The model under review builds one solid part; all positions refer to its coordinate system, in mm. A direction names the side the tool comes from. Coordinates: 2 decimals unless noted, no trailing zeros. Loops run counter-clockwise (first coordinate to the right, second up) from the corner with the lowest first, then second, coordinate; pieces in that order, holes last. Notation, with made-up numbers: M 23,48.25 L 38,48.25 A16 cw 38,56.25 Z; hole C 82.5,68 d5. An arc over 180 degrees is marked long. Use one line per item in the form item = value.
```python
from build123d import *

# Parameters (mm, degrees)
BOSS_EXTRUDE1_DEPTH = 4


with BuildPart() as part:
    # Sketch1 → Boss-Extrude1 (new body)
    with BuildSketch(Plane.XY):
        Polygon((-19, 50), (-19, 5), (-75, 5), (-75, -50), (41, -50), (41, -20), (110, -20), (110, 20), (41, 20), (41, 50), align=None)
        with BuildLine():
            Line((4.364841143, 33.268336331), (4.364841143, -31.161160072))
            ThreePointArc((4.364841143, -31.161160072), (0, -35.526001215), (-4.364841143, -31.161160072))
            Line((-4.364841143, -31.161160072), (-4.364841143, 33.268336331))
            ThreePointArc((-4.364841143, 33.268336331), (0, 37.633177474), (4.364841143, 33.268336331))
        make_face(mode=Mode.SUBTRACT)
        with BuildLine():
            Line((17.594523423, 24.677736811), (17.594523423, -20.257706835))
            ThreePointArc((17.594523423, -20.257706835), (13.229682283, -24.622547975), (8.864841143, -20.257706835))
            Line((8.864841143, -20.257706835), (8.864841143, 24.677736811))
            ThreePointArc((8.864841143, 24.677736811), (13.229682283, 29.042577951), (17.594523423, 24.677736811))
        make_face(mode=Mode.SUBTRACT)
        with BuildLine():
            Line((30.824205703, 12.948264388), (30.824205703, -8.197826739))
            ThreePointArc((30.824205703, -8.197826739), (26.459364563, -12.562667879), (22.094523423, -8.197826739))
            Line((22.094523423, -8.197826739), (22.094523423, 12.948264388))
            ThreePointArc((22.094523423, 12.948264388), (26.459364563, 17.313105528), (30.824205703, 12.948264388))
        make_face(mode=Mode.SUBTRACT)
        with BuildLine():
            Line((-30.824205703, 0.416133702), (-22.094523423, 0.416133702))
            Line((-22.094523423, 0.416133702), (-22.094523423, -10.510680456))
            ThreePointArc((-22.094523423, -10.510680456), (-26.459364563, -14.875521596), (-30.824205703, -10.510680456))
            Line((-30.824205703, -10.510680456), (-30.824205703, 0.416133702))
        make_face(mode=Mode.SUBTRACT)
        with BuildLine():
            Line((-17.594523423, 0.416133702), (-8.864841143, 0.416133702))
            Line((-8.864841143, 0.416133702), (-8.864841143, -24.222598921))
            ThreePointArc((-8.864841143, -24.222598921), (-13.229682283, -28.587440061), (-17.594523423, -24.222598921))
            Line((-17.594523423, -24.222598921), (-17.594523423, 0.416133702))
        make_face(mode=Mode.SUBTRACT)
    extrude(amount=BOSS_EXTRUDE1_DEPTH)


solid = part.part
```
1. Add section A-A (x = 0). State the section outline as (y, z) points, then the cut area to 3 significant figures.
Response values:
outline = M -50,0 L -35.53,0 L -35.53,4 L -50,4 Z; M 37.63,0 L 50,0 L 50,4 L 37.63,4 Z
area = 107 mm^2
2. Add section C-C (y = 43). State the section outline as (x, z) points, then the cut area to 3 significant figures.
Response values:
outline = M -19,0 L 41,0 L 41,4 L -19,4 Z
area = 240 mm^2
3. Insertion check: P1, Ø1.2, axis at y = 37.5, z = 3, coming from the -X side; P2, Ø2, axis at x = 82.5, z = 1.5, coming from the +Y side; P3, Ø6, axis at x = 65.5, y = -1, coming from the -Z side; P4, Ø1.2, axis at x = -44.5, z = 2, coming from the +Y side. Each pin has a flat end and moves straight along its axis. Give the tip position at first contact, or say it passes through.
Response values:
P1 = -19
P2 = 20
P3 = 0
P4 = 5
4. Machinability: for faces 4 (the face through (16, -33, 4)), 5 (the face through (-19, 28, 2)), 6 (the face through (4.365, 2, 2)), 7 (the face through (41, -35, 2)), which of the approach directions +Z, -Z, +X, -X, +Y, -Y give a long, thin tool a straight path to every point of the face, cutting with its end or side? Answer none if there is none.
Response values:
face_4 = +Z, +X, -X, +Y, -Y
face_5 = +Z, -Z, -X, +Y
face_6 = +Z, -Z
face_7 = +Z, -Z, +X, -Y
5. Add section B-B (x = -25.5). State the section outline as (y, z) points, then the cut area to 3 significant figures.
Response values:
outline = M -50,0 L -14.77,0 L -14.77,4 L -50,4 Z; M 0.42,0 L 5,0 L 5,4 L 0.42,4 Z
area = 159 mm^2
6. The part is to be moulded in two halves that separate along X. For faces 1 (the face through (41, 35, 2)), 2 (the face through (-0.096, 37.632, 1.972)), 3 (the face through (-75, -22, 2)), say which applies: pulls with the +X half, pulls with the -X half, needs draft (parallel to the pull), parting line crosses it, or undercut.
Response values:
face_1 = pulls with the +X half
face_2 = undercut
face_3 = pulls with the -X half
7. Wall thickness on line 1 along X through (y, z) = (-4, 0.8); line 2 along X through (y, z) = (-27, 0.8); line 3 along X through (y, z) = (-27.5, 1.15): over which ranges is each line inside the solid? List them lowest first. Write a range as from..to.
Response values:
line_1 = -75..-30.82, -22.09..-17.59, -8.86..-4.36, 4.36..8.86, 17.59..22.09, 30.82..110
line_2 = -75..-16.6, -9.86..-4.36, 4.36..41
line_3 = -75..-16.11, -10.35..-4.36, 4.36..41
8. Add section D-D (x = 58.5). State the section outline as (y, z) points.
Response values:
outline = M -20,0 L 20,0 L 20,4 L -20,4 Z
